```python
from build123d import *

# Parameters (mm, degrees)
F1_DEPTH      = 5.6
F1_DEPTH_BACK = 5.6
F2_DEPTH      = 3.1
F2_DEPTH_BACK = 3.1
F0_W          = 2.5
F0_H          = 11.875
F3_DEPTH      = 1.2
F3_DEPTH_BACK = 3.1
F4_DEPTH      = 5
F4_DEPTH_BACK = 5


with BuildPart() as f1:
    # F0 (on Front) → F1 (new body, two sides)
    with BuildSketch(Plane.XZ) as f1_sk:
        Polygon((2.5, -11.875), (0, -11.875), (0, -23.125), (2.5, -23.125), (30, -23.125), (30, -11.875), align=None)
    extrude(amount=F1_DEPTH)
    extrude(f1_sk.sketch, amount=-F1_DEPTH_BACK)

    # F0 (on Front) → F2 (join, two sides)
    with BuildSketch(Plane.XZ) as f2_sk:
        Polygon((27.4, 0), (2.5, 0), (2.5, -11.875), (30, -11.875), (34.6922105263, -6.9), (27.4, -6.9), align=None)
        with BuildLine():
            ThreePointArc((9.7, -5.6), (10.3443650814, -4.0443650814), (11.9, -3.4))
            Line((11.9, -3.4), (21.3, -3.4))
            ThreePointArc((21.3, -3.4), (22.8556349186, -4.0443650814), (23.5, -5.6))
            ThreePointArc((23.5, -5.6), (22.8556349186, -7.1556349186), (21.3, -7.8))
            Line((21.3, -7.8), (11.9, -7.8))
            ThreePointArc((11.9, -7.8), (10.3443650814, -7.1556349186), (9.7, -5.6))
        make_face(mode=Mode.SUBTRACT)
        Polygon((30, -23.125), (2.5, -23.125), (2.5, -35), (27.4, -35), (27.4, -28.1), (34.6922105263, -28.1), align=None)
        with BuildLine():
            ThreePointArc((11.9, -31.6), (10.3443650814, -30.9556349186), (9.7, -29.4))
            ThreePointArc((9.7, -29.4), (10.3443650814, -27.8443650814), (11.9, -27.2))
            Line((11.9, -27.2), (21.3, -27.2))
            ThreePointArc((21.3, -27.2), (22.8556349186, -27.8443650814), (23.5, -29.4))
            ThreePointArc((23.5, -29.4), (22.8556349186, -30.9556349186), (21.3, -31.6))
            Line((21.3, -31.6), (11.9, -31.6))
        make_face(mode=Mode.SUBTRACT)
    extrude(amount=F2_DEPTH)
    extrude(f2_sk.sketch, amount=-F2_DEPTH_BACK)

    # F0 (on Front) → F3 (join, two sides)
    with BuildSketch(Plane.XZ) as f3_sk:
        with Locations((1.25, -5.9375)):
            Rectangle(F0_W, F0_H)
        with Locations((1.25, -29.0625)):
            Rectangle(F0_W, F0_H)
    extrude(amount=F3_DEPTH)
    extrude(f3_sk.sketch, amount=-F3_DEPTH_BACK)

    # F0 (on Front) → F4 (join, two sides)
    with BuildSketch(Plane.XZ) as f4_sk:
        Polygon((41.2, 0), (27.4, 0), (27.4, -6.9), (34.6922105263, -6.9), align=None)
        Polygon((41.2, -35), (34.6922105263, -28.1), (27.4, -28.1), (27.4, -35), align=None)
    extrude(amount=F4_DEPTH)
    extrude(f4_sk.sketch, amount=-F4_DEPTH_BACK)


solid = f1.part
```
Design review of the part built by this model. Coordinates are the model's own, in mm. A direction names the side the tool comes from. Give positions to 0.01 mm unless a question says otherwise; leave off trailing zeros. Write each loop counter-clockwise with the first axis right and the second up, starting at its lowest first coordinate (ties: lowest second). Pieces come first, ordered by that corner, then holes. Notation, with made-up numbers: (-15.5, 40.5) - (8.5, 40.5) arc R19 cw to (8.5, 71.5) - close; hole circle Ø9 at (79, -7). An arc over 180 degrees is marked (long way). Return JSON: item names as keys, results as strings. Group by question number.
(1) Insertion check: pin 1 (1.5 mm diameter, centred on y = -3, z = -17, fed in from +X); pin 2 (9.5 mm diameter, centred on x = 18.5, z = -6, fed in from +Y); pin 3 (2 mm diameter, centred on x = 32.5, z = -2.5, fed in from -Y). Each pin has a flat end and moves straight along its axis. Give the tip position at first contact, or say it passes through.
(2) Machinability: for faces 1 (the flat face through (31, 4, -28.1)), 2 (the flat face through (17, 0, -3.4)), 3 (the flat face through (27.4, -4, -32)), 4 (the flat face through (1, -1.2, -6)), 5 (the flat face through (27.4, 4, -3)), which of the approach directions +Z, -Z, +X, -X, +Y, -Y give a long, thin tool a straight path to every point of the face, cutting with its end or side? Answer none if there is none.
(3) We need section B-B, the plane x = 35.5. Give the boundary of the cut face in (y, z).
(4) Mouldability with a two-part tool opening along X and no side actions: class faces 6 (the flat face through (2.5, -2, -29)), 7 (the flat face through (31, 4, -6.9)), 8 (the flat face through (17, 0, -27.2)) as +X half, -X half, draft (parallel to the pull), parting line (faces both ways), or undercut.
(5) We need section A-A, the plane y = -4.5. Give the boundary of the cut face in (x, z) (3 decimals).
(6) We need section C-C, the plane y = 1.25. Give the boundary of the cut face in (x, z) (3 decimals).
(7) We need section D-D, the plane x = 6. Give the boundary of the cut face in (y, z) (3 decimals).
(8) To check wall thickness, follow probe 1 along Z at (x, y) = (28, 4) (3 decimals); probe 2 along Z at (x, y) = (18, -2.25); probe 3 along Z at (x, y) = (32, -3.5). State the ranges of each line that lie inside material, in increasing order.
Reported:
{
 "1": {"pin 1": "stops at x = 30", "pin 2": "stops at y = 3.1", "pin 3": "stops at y = -5"},
 "2": {"face 1": "+X, -X, +Y", "face 2": "+Y, -Y", "face 3": "-Z, -X, -Y", "face 4": "+Z, -X, -Y", "face 5": "+Z, -X, +Y"},
 "3": {"outline": "(-5, -35) - (5, -35) - (5, -28.96) - (-5, -28.96) - close; (-5, -6.04) - (5, -6.04) - (5, 0) - (-5, 0) - close"},
 "4": {"face 6": "-X half", "face 7": "draft", "face 8": "undercut"},
 "5": {"outline": "(0, -23.125) - (30, -23.125) - (30, -11.875) - (0, -11.875) - close; (27.4, -35) - (41.2, -35) - (34.692, -28.1) - (27.4, -28.1) - close; (27.4, -6.9) - (34.692, -6.9) - (41.2, 0) - (27.4, 0) - close"},
 "6": {"outline": "(0, -35) - (41.2, -35) - (30, -23.125) - (30, -11.875) - (41.2, 0) - (0, 0) - close; hole (11.9, -31.6) - (21.3, -31.6) arc R2.2 ccw to (21.3, -27.2) - (11.9, -27.2) arc R2.2 ccw to start; hole (11.9, -7.8) - (21.3, -7.8) arc R2.2 ccw to (21.3, -3.4) - (11.9, -3.4) arc R2.2 ccw to start"},
 "7": {"outline": "(-5.6, -23.125) - (-3.1, -23.125) - (-3.1, -35) - (3.1, -35) - (3.1, -23.125) - (5.6, -23.125) - (5.6, -11.875) - (3.1, -11.875) - (3.1, 0) - (-3.1, 0) - (-3.1, -11.875) - (-5.6, -11.875) - close"},
 "8": {"probe 1": "z = -35 to -28.1, -23.125 to -11.875, -6.9 to 0", "probe 2": "z = -35 to -31.6, -27.2 to -7.8, -3.4 to 0", "probe 3": "z = -35 to -28.1, -6.9 to 0"}
}
